Geometry check sheet. Reference: the model listing, model coordinates, mm. A direction names the side the tool comes from. Give positions to 0.01 mm unless a question says otherwise; leave off trailing zeros. Write each loop counter-clockwise with the first axis right and the second up, starting at its lowest first coordinate (ties: lowest second). Pieces come first, ordered by that corner, then holes. Notation, with made-up numbers: (19.5, 72.5) - (44.5, 72.5) arc R27 ccw to (44.5, 98.5) - close; hole circle Ø3 at (26.5, 10.25). An arc over 180 degrees is marked (long way). One line per question, with ' | ' between items. Start each with the question number.
Q1. Section check C-C on y = 5. Record the boundary of the cut face in (x, z), and give its area (3 significant figures).
Q2. Section check B-B on z = 2. Count the separate pieces of the cut face and the enclosed holes in it, and give its area (3 significant figures).
Q3. Release check for a two-part mould opening along Y. For faces 4 (the face through (27, 15, 10)), 5 (the face through (13, 6, 2)), 6 (the face through (14, 18, 15)) record: +Y half, -Y half, draft (parallel to the pull), parting line (faces both ways), or undercut.
Q4. Section check A-A on x = 5. Record the boundary of the cut face in (y, z), and give its area (3 significant figures).
Q5. Set-up check for faces 1 (the face through (33.89, 31.01, 3.03)), 2 (the face through (12.5, 5, 2)), 3 (the face through (34.5, 17.5, 9.9)): record each of +Z, -Z, +X, -X, +Y, -Y from which the full face is reachable in a straight line by a thin tool's end or side.
Q6. Thickness scan on L1, parallel to X at y = 5, z = 0.85; L2, parallel to Y at x = 35, z = 3.6; L3, parallel to X at y = 30, z = 4. Record the ranges inside material, lowest first. Write a range as [from, to].
Q7. Section check D-D on z = 11.75. Record the boundary of the cut face in (x, y).
Q8. Gauge pin test, flat ends, axial feed: P1, Ø8, axis at y = 28, z = 2, coming from the -X side; P2, Ø1.1, axis at x = 35, z = 8.5, coming from the +Y side; P3, Ø3, axis at y = 12, z = 9.5, coming from the -X side; P4, Ø3, axis at x = 26.5, y = 30, coming from the +Z side. Record the tip position at first contact, or that the pin passes through.
Autodesk Inventor part; units mm, degrees
ref_plane "YZ Plane" through (0, 0, 0) normal (1, 0, 0) x (0, 1, 0)
ref_plane "XZ Plane" through (0, 0, 0) normal (0, 1, 0) x (-1, 0, 0)
ref_plane "XY Plane" through (0, 0, 0) normal (0, 0, 1) x (1, 0, 0)
sketch "Эскиз1" plane through (0, 0, 0) normal (0, 0, 1) x (1, 0, 0)
  line L0 (0, 0) -> (40, 0)
  line L1 (40, 0) -> (40, 35)
  line L2 (40, 35) -> (0, 35)
  line L3 (0, 35) -> (0, 0)
  line L4 (0, 17.5) -> (40, 17.5)
  line L5 (5, 5) -> (35, 5)
  line L6 (35, 5) -> (35, 30)
  line L7 (35, 30) -> (5, 30)
  line L8 (5, 30) -> (5, 5)
  line L9 (5, 5) -> (35, 30) construction
  line L10 (35, 5) -> (5, 30) construction
  circle A0 centre (5, 30) radius 2.5
  line L11 (5, 30) -> (14, 30)
  circle A1 centre (14, 30) radius 1.5
  line L12 (2.5, 2.5) -> (7.5, 2.5)
  line L13 (7.5, 2.5) -> (7.5, 7.5)
  line L14 (7.5, 7.5) -> (2.5, 7.5)
  line L15 (2.5, 7.5) -> (2.5, 2.5)
  line L16 (2.5, 2.5) -> (7.5, 7.5) construction
  line L17 (7.5, 2.5) -> (2.5, 7.5) construction
  line L18 (5, 5) -> (13.5, 5)
  line L19 (12.5, 6) -> (14.5, 6)
  line L20 (14.5, 6) -> (14.5, 4)
  line L21 (14.5, 4) -> (12.5, 4)
  line L22 (12.5, 4) -> (12.5, 6)
  line L23 (12.5, 6) -> (14.5, 4) construction
  line L24 (14.5, 6) -> (12.5, 4) construction
  point P0 (20, 17.5)
  dimension "d0" = 40
  dimension "d1" = 35
  dimension "d2" = 30
  dimension "d3" = 25
  dimension "d4" = 5
  dimension "d5" = 9
  dimension "d6" = 3
  dimension "d7" = 5
  dimension "d8" = 5
  dimension "d9" = 8.5
  dimension "d10" = 2
  dimension "d11" = 2
extrude "Выдавливание1" add sketch "Эскиз1" along normal blind 5 contours L3 L4 L8 L14 L15 L12 L13 L5 L22 L21 L20 L6 L1 L0 | L3 L2 L1 L4 L6 L7 A1 A0 L8 | L8 A0 L7 A1 L6 L4 | L4 L6 L5 L20 L19 L22 L13 L14 L8
sketch "Эскиз3" plane through (0, 0, 5) normal (0, 0, 1) x (1, 0, 0)
  line L0 (0, 35) -> (0, 0)
  line L1 (0, 17.5) -> (40, 17.5)
  line L2 (40, 0) -> (40, 35)
  line L3 (40, 0) -> (40, 35)
  line L4 (40, 35) -> (0, 35)
  line L5 (0, 35) -> (0, 0)
  line L6 (0, 0) -> (40, 0)
  line L7 (7.5, 7.5) -> (7.5, 2.5)
  line L8 (7.5, 2.5) -> (2.5, 2.5)
  line L9 (2.5, 2.5) -> (2.5, 7.5)
  line L10 (2.5, 7.5) -> (7.5, 7.5)
  line L11 (14.5, 4) -> (12.5, 4)
  line L12 (12.5, 4) -> (12.5, 6)
  line L13 (12.5, 6) -> (14.5, 6)
  line L14 (14.5, 6) -> (14.5, 4)
  circle A0 centre (14, 30) radius 1.5
  circle A1 centre (5, 30) radius 2.5
  line L15 (5, 5) -> (35, 5)
  line L16 (35, 5) -> (35, 30)
  line L17 (35, 30) -> (5, 30)
  line L18 (5, 30) -> (5, 5)
  line L19 (5, 5) -> (35, 30) construction
  line L20 (35, 5) -> (5, 30) construction
  line L21 (34.5, 17) -> (35.5, 17)
  line L22 (35.5, 17) -> (35.5, 18)
  line L23 (35.5, 18) -> (34.5, 18)
  line L24 (34.5, 18) -> (34.5, 17)
  line L25 (34.5, 17) -> (35.5, 18) construction
  line L26 (35.5, 17) -> (34.5, 18) construction
  line L27 (35, 17.5) -> (27, 17.5)
  line L28 (24.5, 15) -> (29.5, 15)
  line L29 (29.5, 15) -> (29.5, 20)
  line L30 (29.5, 20) -> (24.5, 20)
  line L31 (24.5, 20) -> (24.5, 15)
  line L32 (24.5, 15) -> (29.5, 20) construction
  line L33 (29.5, 15) -> (24.5, 20) construction
  line L34 (27, 17.5) -> (14.5, 17.5)
  line L35 (9.5, 12.5) -> (19.5, 12.5)
  line L36 (19.5, 12.5) -> (19.5, 22.5)
  line L37 (19.5, 22.5) -> (9.5, 22.5)
  line L38 (9.5, 22.5) -> (9.5, 12.5)
  line L39 (9.5, 12.5) -> (19.5, 22.5) construction
  line L40 (19.5, 12.5) -> (9.5, 22.5) construction
  line L41 (24.5, 20) -> (29.5, 20)
  line L42 (29.5, 20) -> (29.5, 15)
  line L43 (29.5, 15) -> (24.5, 15)
  line L44 (24.5, 15) -> (24.5, 20)
  point P0 (20, 17.5)
  dimension "d14" = 35
  dimension "d15" = 40
  dimension "d16" = 30
  dimension "d17" = 25
  dimension "d18" = 1
  dimension "d19" = 1
  dimension "d20" = 8
  dimension "d21" = 5
  dimension "d22" = 5
  dimension "d23" = 12.5
  dimension "d24" = 10
  dimension "d25" = 10
extrude "Выдавливание2" add sketch "Эскиз3" along normal blind 10 contours L38 L37 L36 L1 | L1 L36 L35 L38 | L22 L21 L16 L1 | L1 L16 L23 L22 | L16 L21 L24 L1 | L1 L24 L23 L16 | L31 L30 L29 L1 | L1 L29 L28 L31
sketch "Эскиз4" plane through (0, 0, 5) normal (0, 0, 1) x (1, 0, 0)
  line L0 (34.5, 17) -> (34.5, 18)
  line L1 (34.5, 18) -> (35.5, 18)
  line L2 (35.5, 18) -> (35.5, 17)
  line L3 (35.5, 17) -> (34.5, 17)
  line L4 (19.5, 22.5) -> (19.5, 12.5)
  line L5 (19.5, 12.5) -> (9.5, 12.5)
  line L6 (9.5, 12.5) -> (9.5, 22.5)
  line L7 (9.5, 22.5) -> (19.5, 22.5)
  line L8 (24.5, 15) -> (24.5, 20)
  line L9 (24.5, 20) -> (29.5, 20)
  line L10 (29.5, 20) -> (29.5, 15)
  line L11 (29.5, 15) -> (24.5, 15)
  line L12 (0, 35) -> (0, 0)
  line L13 (0, 0) -> (40, 0)
  line L14 (40, 0) -> (40, 35)
  line L15 (40, 35) -> (0, 35)
  line L16 (2.5, 2.5) -> (2.5, 7.5)
  line L17 (2.5, 7.5) -> (7.5, 7.5)
  line L18 (7.5, 7.5) -> (7.5, 2.5)
  line L19 (7.5, 2.5) -> (2.5, 2.5)
  line L20 (12.5, 6) -> (14.5, 6)
  line L21 (14.5, 6) -> (14.5, 4)
  line L22 (14.5, 4) -> (12.5, 4)
  line L23 (12.5, 4) -> (12.5, 6)
  circle A0 centre (14, 30) radius 1.5
  circle A1 centre (5, 30) radius 2.5
  line L24 (0, 35) -> (0, 0)
  line L25 (0, 17.5) -> (40, 17.5)
  line L26 (40, 0) -> (40, 35)
  line L27 (5, 5) -> (35, 5)
  line L28 (35, 5) -> (35, 30)
  line L29 (35, 30) -> (5, 30)
  line L30 (5, 30) -> (5, 5)
  line L31 (5, 5) -> (35, 30) construction
  line L32 (35, 5) -> (5, 30) construction
  circle A2 centre (35, 30) radius 1.5
  line L33 (35, 30) -> (26.5, 30)
  circle A3 centre (26.5, 30) radius 2
  circle A4 centre (35, 5) radius 2.5
  line L34 (35, 5) -> (24, 5)
  circle A5 centre (24, 5) radius 3.5
  point P0 (20, 17.5)
  dimension "d28" = 30
  dimension "d29" = 25
  dimension "d30" = 35
  dimension "d31" = 40
  dimension "d32" = 3
  dimension "d33" = 8.5
  dimension "d34" = 4
  dimension "d35" = 5
  dimension "d36" = 11
  dimension "d37" = 7
extrude "Выдавливание3" cut sketch "Эскиз4" against normal blind 4 contours A4 L27 L28 | L28 L27 A4 | A2 L29 L28 | L28 L29 A2 | A5 L27 | L27 A5 | A3 L29 | L29 A3
sketch "Эскиз5" plane through (26.5, 30, 1) normal (0, 0, 1) x (1, 0, 0)
  circle A0 centre (0, 0) radius 2
  circle A1 centre (8.5, 0) radius 1.5
  circle A2 centre (-2.5, -25) radius 3.5
  circle A3 centre (8.5, -25) radius 2.5
  point P0 (-26.5, -30)
hole "Отверстие1" at (26.5, 30, 1) at (35, 30, 1) at (24, 5, 1) at (35, 5, 1) direction (0, 0, -1) diameter 2 end through all
properties part number "Тестовая модель (Валы, столбы, подшипники)"
Working result:
1) outline: (0, 0) - (2.5, 0) - (2.5, 5) - (0, 5) - close; (7.5, 0) - (12.5, 0) - (12.5, 5) - (7.5, 5) - close; (14.5, 0) - (23, 0) - (23, 1) - (20.5, 1) - (20.5, 5) - (14.5, 5) - close; (25, 0) - (34, 0) - (34, 1) - (32.5, 1) - (32.5, 5) - (27.5, 5) - (27.5, 1) - (25, 1) - close; (36, 0) - (40, 0) - (40, 5) - (37.5, 5) - (37.5, 1) - (36, 1) - close | area: 113 mm2
2) separate pieces: 1 | enclosed holes: 8 | area: 1,270 mm2
3) face 4: -Y half | face 5: undercut | face 6: draft
4) outline: (0, 0) - (2.5, 0) - (2.5, 5) - (0, 5) - close; (7.5, 0) - (27.5, 0) - (27.5, 5) - (7.5, 5) - close; (32.5, 0) - (35, 0) - (35, 5) - (32.5, 5) - close | area: 125 mm2
5) face 1: +Z | face 2: +Z, -Z | face 3: +Z, +Y, -Y
6) L1: x = [0, 2.5], [7.5, 12.5], [14.5, 23], [25, 34], [36, 40] | L2: y = [0, 2.5], [7.5, 28.5], [31.5, 35] | L3: x = [0, 2.5], [7.5, 12.5], [15.5, 24.5], [28.5, 33.5], [36.5, 40]
7) outline: (9.5, 12.5) - (19.5, 12.5) - (19.5, 22.5) - (9.5, 22.5) - close; (24.5, 15) - (29.5, 15) - (29.5, 20) - (24.5, 20) - close; (34.5, 17) - (35.5, 17) - (35.5, 18) - (34.5, 18) - close
8) P1: stops at x = 0 | P2: stops at y = 18 | P3: stops at x = 9.5 | P4: stops at z = 1
